from build123d import *

# Parameters (mm, degrees)
ESQUISSE1_R        = 3.9
BOSS_EXTRU_1_DEPTH = 9
CONG_1_R           = 3.9
BOSS_EXTRU_2_DEPTH = 2
ESQUISSE3_W        = 0.6
ESQUISSE3_H        = 0.6
BOSS_EXTRU_3_DEPTH = 6.8
ESQUISSE6_W        = 0.6
ESQUISSE6_H        = 0.6
BOSS_EXTRU_4_DEPTH = 7
ESQUISSE8_W        = 0.6
ESQUISSE8_H        = 0.6
BOSS_EXTRU_5_DEPTH = 7


with BuildPart() as part:
    # Esquisse1 → Boss.-Extru.1 (new body)
    with BuildSketch(Plane(origin=(0, 0, 0), x_dir=(1, 0, 0), z_dir=(0, 1, 0))):
        Circle(ESQUISSE1_R)
    extrude(amount=BOSS_EXTRU_1_DEPTH)

    # Congé1
    cong_1_edges = [part.edges().sort_by_distance(p)[0] for p in [
        (-3.9, 9, 0),
    ]]
    fillet(cong_1_edges, radius=CONG_1_R)

    # Esquisse2 → Boss.-Extru.2 (add)
    with BuildSketch(Plane.XZ):
        with BuildLine():
            Line((2.343608329, 3.9), (-2.343608329, 3.9))
            ThreePointArc((-2.343608329, 3.9), (0, -4.55), (2.343608329, 3.9))
        make_face()
    extrude(amount=BOSS_EXTRU_2_DEPTH)

    # Esquisse3 → Boss.-Extru.3 (add)
    with BuildSketch(Plane.XZ.offset(2)):
        with Locations((0, 0.275)):
            Rectangle(ESQUISSE3_W, ESQUISSE3_H)
        with Locations((0, -0.925)):
            Rectangle(ESQUISSE3_W, ESQUISSE3_H)
    extrude(amount=BOSS_EXTRU_3_DEPTH)

    # Esquisse6 → Boss.-Extru.4 (add)
    with BuildSketch(Plane(origin=(0, -2.123198642, 0.298396109), x_dir=(-1, 0, 0), z_dir=(0, -0.990268069, 0.139173101))):
        with Locations((0, -1.185218779)):
            Rectangle(ESQUISSE6_W, ESQUISSE6_H)
    extrude(amount=BOSS_EXTRU_4_DEPTH)

    # Esquisse8 → Boss.-Extru.5 (add)
    with BuildSketch(Plane(origin=(0, -2.212780783, -0.310986058), x_dir=(-1, 0, 0), z_dir=(0, -0.990268069, -0.139173101))):
        with Locations((0, 1.828893024)):
            Rectangle(ESQUISSE8_W, ESQUISSE8_H)
    extrude(amount=BOSS_EXTRU_5_DEPTH)


solid = part.part
Read the model definition and answer for the solid it produces. Units are mm, in the model's axes. A direction names the side the tool comes from. Give positions to 0.01 mm unless a question says otherwise; leave off trailing zeros. Write each loop counter-clockwise with the first axis right and the second up, starting at its lowest first coordinate (ties: lowest second). Pieces come first, ordered by that corner, then holes. Notation, with made-up numbers: (-16.75, 37) - (37.25, 37) arc R27 cw to (37.25, 73) - close; hole circle Ø3 at (54, -33). An arc over 180 degrees is marked (long way). Return JSON: item names as keys, results as strings.
Q1. For a pull along Z with two mould halves and no side action, classify faces 6 (the face through (0.004, -5.376, -2.905)), 7 (the face through (0.3, -5, 2)), 8 (the face through (0.004, -5.376, 2.255)), 9 (the face through (0.004, -5.417, 1.655)) as released by +Z, released by -Z, zero draft, split by the parting line, or undercut.
Reply:
{"face 6": "released by -Z", "face 7": "zero draft", "face 8": "released by +Z", "face 9": "undercut"}
Q2. Given P1, Ø2, axis at y = 6, z = 1, coming from the -X side; P2, Ø1, axis at x = -1, z = 0.5, coming from the -Y side; P3, Ø0.8, axis at y = -4, z = 2, coming from the +X side; P4, Ø4, axis at x = -2.5, y = -5, coming from the -Z side (3 decimals), each flat-ended and moving along its own axis, determine where each tip first touches the part or whether it passes through.
Reply:
{"P1": "x = -3.88", "P2": "y = -2", "P3": "x = 0.3", "P4": "through"}
Q3. A cutting plane is placed at D-D, the plane z = -1.5. Determine the outline of the cut face in (x, y), and give its area (3 significant figures).
Reply:
{"outline": "(-4.3, -2) - (4.3, -2) - (4.3, 0) - (3.6, 0) - (3.6, 5.1) arc R3.6 ccw to (-3.6, 5.1) - (-3.6, 0) - (-4.3, 0) - close", "area": "74.3 mm²"}
Q4. Consider line 1 along X through (y, z) = (3.5, 0); line 2 along X through (y, z) = (-6, 2); line 3 along Y through (x, z) = (-3, 1.75). Determine where each line is inside the solid, lowest interval first. Write a range as [from, to].
Reply:
{"line 1": "[-3.9, 3.9]", "line 2": "[-0.3, 0.3]", "line 3": "[-2, 6.87]"}
Q5. A cutting plane is placed at A-A, the plane z = -3. Determine the outline of the cut face in (x, y), and give its area (3 significant figures).
Reply:
{"outline": "(-3.42, -2) - (3.42, -2) - (3.42, 0) - (2.49, 0) - (2.49, 5.1) arc R2.49 ccw to (-2.49, 5.1) - (-2.49, 0) - (-3.42, 0) - close; (-0.3, -8.9) - (0.3, -8.9) - (0.3, -6.05) - (-0.3, -6.05) - close", "area": "50.6 mm²"}
Q6. For faces 1 (the face through (-2.87, 2.51, -2.64)), 2 (the face through (-0.3, -5.4, -2.6)), 3 (the face through (0.004, -5.417, -2.305)), 4 (the face through (0, -1, 3.9)), 5 (the face through (0.3, -5.4, -2.6)), determine the directions among +Z, -Z, +X, -X, +Y, -Y from which every point of the face is accessible in a straight line to the end or side of a thin tool.
Reply:
{"face 1": "+Y", "face 2": "+Z, -Z, -X, -Y", "face 3": "+X, -X, -Y", "face 4": "+Z, +X, -X, +Y, -Y", "face 5": "+Z, -Z, +X, -Y"}
Q7. A cutting plane is placed at C-C, the plane x = -3.5. Determine the outline of the cut face in (y, z).
Reply:
{"outline": "(-2, -2.91) - (0, -2.91) - (0, -1.72) - (5.1, -1.72) arc R1.72 ccw to (5.1, 1.72) - (0, 1.72) - (0, 2.91) - (-2, 2.91) - close"}
Q8. A cutting plane is placed at B-B, the plane y = -3.75. Determine the outline of the cut face in (x, z) (3 decimals).
Reply:
{"outline": "(-0.3, -2.677) - (0.3, -2.677) - (0.3, -2.071) - (-0.3, -2.071) - close; (-0.3, -1.225) - (0.3, -1.225) - (0.3, -0.625) - (-0.3, -0.625) - close; (-0.3, -0.025) - (0.3, -0.025) - (0.3, 0.575) - (-0.3, 0.575) - close; (-0.3, 1.421) - (0.3, 1.421) - (0.3, 2.027) - (-0.3, 2.027) - close"}
